Model file for the job. Use its own axes, mm. A direction names the side the tool comes from. Give positions to 0.01 mm unless a question says otherwise; leave off trailing zeros. Order: outer loops, then holes, each group sorted by start corner. A loop starts at its lowest first (then second) coordinate and runs counter-clockwise, first axis right, second up. Notation, with made-up numbers: (19, 71) - (45, 71) arc R20 ccw to (45, 90) - close; hole circle Ø11 at (42, 72). An arc over 180 degrees is marked (long way). Use CSV: the item, a comma, the result in double quotes. Start each with the question number.
(1) Band-saw the part on D-D, the plane z = 1. Give the cut face in (x, y).
(2) Band-saw the part on B-B, the plane y = -0.5. Give the cut face in (x, z).
(3) Drop flat-ended pins along their axis: pin 1 Ø1 at (x, z) = (-3, 12.5) entering from +Y; pin 2 Ø5 at (x, z) = (-4, 12) entering from -Y. Give the stop position or say it passes through.
(4) Band-saw the part on C-C, the plane x = 3.5. Give the cut face in (y, z), then the cut area to 3 significant figures.
(5) Band-saw the part on A-A, the plane x = 2.25. Give the cut face in (y, z), then the cut area to 3 significant figures.
(6) Probe L1, parallel to Y at x = 2.25, z = 10.25; L2, parallel to Z at x = -1.75, y = -2.75; L3, parallel to Y at x = 2, z = 9. List the from-to ranges inside material, lowest first.
(7) Pull direction Y, two halves, no side cores. Call faces 4 (the flat face through (1.75, 4.446, 7.605)), 5 (the flat face through (0, 0, 0)): +Y half, -Y half, draft (parallel to the pull), parting line (faces both ways), or undercut.
(8) Tool access for faces 1 (the cylindrical face through (-1.26, 3.81, 8.59)), 2 (the flat face through (2.121, 4.194, 7.605)), 3 (the flat face through (0, -2, 15)): list every direction of +Z, -Z, +X, -X, +Y, -Y with a clear straight run to the whole face (end or side of a thin tool).
Autodesk Fusion 360 part; units mm, degrees
sketch "Sketch2" plane through (0, 0, 0) normal (0, 0, 1) x (1, 0, 0) in component "2x12AWG_silicone, 1x DS18B"
  circle A0 centre (0, 0) radius 5.5
  dimension "d8" = 11
extrude "Extrude1" add sketch "Sketch2" along normal blind 15 in component "2x12AWG_silicone, 1x DS18B"
sketch "Sketch3" plane through (0, 0, 15) normal (0, 0, 1) x (-1, 0, 0) in component "2x12AWG_silicone, 1x DS18B"
  circle A0 centre (0, 0) radius 5.5
  circle A1 centre (2.25, 0.9695) radius 2.25
  circle A2 centre (-2.25, 0.9695) radius 2.25
  circle A3 centre (0, -2.4579) radius 1.85
  circle A4 centre (0, 0) radius 4.7 construction
  dimension "d11" = 4.5
  dimension "d12" = 3.7
  dimension "d13" = 0.8
extrude "Extrude2" cut sketch "Sketch3" against normal blind 13 contours A1 | A2 | A1 A2 A3 | A3 in component "2x12AWG_silicone, 1x DS18B"
fillet "Fillet1" radius 0.2 3 edges at (-1.0152, 0.9114, 8.5) (0, -0.9695, 8.5) (1.0152, 0.9114, 8.5) in component "2x12AWG_silicone, 1x DS18B"
sketch "Sketch4" plane through (0, 0, 15) normal (0, 0, 1) x (-1, 0, 0) in component "2x12AWG_silicone, 1x DS18B"
  arc A0 (-1.6028, -1.5341) -> (-1.8148, -1.238) centre (-1.7761, -1.4342) ccw
  arc A1 (-0.1837, 1.8599) -> (-1.8148, -1.238) centre (-2.25, 0.9695) ccw
  arc A2 (-0.1837, 1.8599) -> (0.1837, 1.8599) centre (0, 1.9391) ccw
  arc A3 (1.8148, -1.238) -> (0.1837, 1.8599) centre (2.25, 0.9695) ccw
  arc A4 (1.8148, -1.238) -> (1.6028, -1.5341) centre (1.7761, -1.4342) ccw
  arc A5 (-1.6028, -1.5341) -> (1.6028, -1.5341) centre (0, -2.4579) ccw
  circle A6 centre (0, 0) radius 5.5
  line L0 (-0.9824, -4.0255) -> (-2.539, -4.8789)
  line L1 (-1.3198, -3.7543) -> (-2.9449, -4.6452)
  dimension "d18" = 0.4
extrude "Extrude3" cut sketch "Sketch4" against normal blind 16.5 contours A5 A6 L0 L1 in component "2x12AWG_silicone, 1x DS18B"
component "2x12AWG_silicone, 1x DS18B" placed x (1, 0, 0) y (0, 1, 0) z (0, 0, 1) at (0, 0, 0)
equation "Si12AWG = 4.6 mm"
equation "DS18B20 = 3.7 mm"
equation "clearance = 0.2 mm"
equation "gland_ID_max = 12 mm"
equation "gland_ID_min = 5.65 mm"
equation "insert_D = 9 mm"
equation "insert_L = 15 mm"
equation "d8 = gland_ID_max - 1 mm"
equation "d9 = insert_L"
equation "d11 = Si12AWG - clearance / 2"
equation "d12 = DS18B20"
Answer block:
1,outline,"(0.98, 4.03) - (2.54, 4.88) arc R5.5 ccw (long way) to (2.94, 4.65) - (1.32, 3.75) arc R1.85 ccw to start"
2,outline,"(-5.48, 0) - (5.48, 0) - (5.48, 15) - (4.45, 15) - (4.45, 2) - (-4.45, 2) - (-4.45, 15) - (-5.48, 15) - close"
3,pin 1,"stops at y = 4.9"
3,pin 2,"stops at y = -5.29"
4,outline,"(-4.24, 0) - (4.24, 0) - (4.24, 15) - (0.9, 15) - (0.9, 2) - (-2.84, 2) - (-2.84, 15) - (-4.24, 15) - close"
4,area,"78.6 mm2"
5,outline,"(-5.02, 0) - (4.26, 0) - (4.26, 15) - (1.28, 15) - (1.28, 2) - (-3.22, 2) - (-3.22, 15) - (-5.02, 15) - close; (4.72, 0) - (5.02, 0) - (5.02, 15) - (4.72, 15) - close"
5,area,"85.2 mm2"
6,L1,"y = -5.02 to -3.22, 1.28 to 4.26, 4.72 to 5.02"
6,L2,"z = 0 to 2"
6,L3,"y = -5.12 to -3.21, 1.27 to 4.13, 4.58 to 5.12"
7,face 4,"undercut"
7,face 5,"draft"
8,face 1,"+Z"
8,face 2,"+Z, -Z"
8,face 3,"+Z, +X, -X, +Y, -Y"
